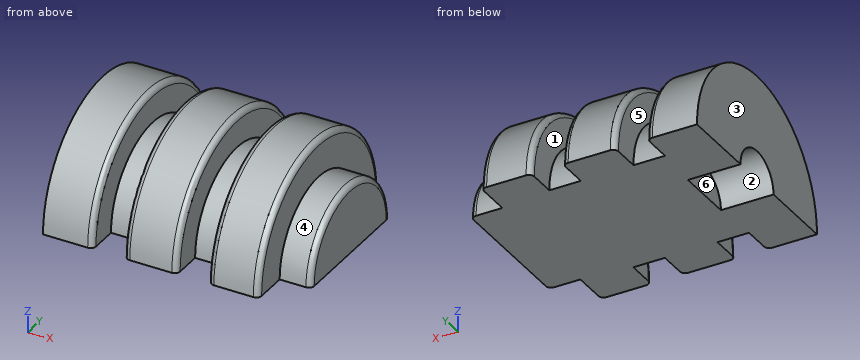
```python
from build123d import *

# Parameters (mm, degrees)
SKETCH1_R           = 10
BOSS_EXTRUDE1_DEPTH = 4.75
SKETCH4_R           = 6.5
BOSS_EXTRUDE2_DEPTH = 3
SKETCH5_R           = 7
BOSS_EXTRUDE3_DEPTH = 3
FILLET1_R           = 0.5
BOSS_EXTRUDE4_START = 5
SKETCH6_R           = 10
BOSS_EXTRUDE4_DEPTH = 5
SKETCH7_R           = 7
BOSS_EXTRUDE5_DEPTH = 3
BOSS_EXTRUDE6_START = 4.75
SKETCH9_R           = 10
BOSS_EXTRUDE6_DEPTH = 4.75
FILLET2_R           = 0.5
SKETCH10_W          = 23.933386236
SKETCH10_H          = 20
CUT_EXTRUDE1_DEPTH  = 20
CUT_EXTRUDE2_DEPTH  = 5


with BuildPart() as part:
    # Sketch1 → Boss-Extrude1 (new body)
    with BuildSketch(Plane(origin=(0, 0, 0), x_dir=(0, 0, -1), z_dir=(1, 0, 0))):
        Circle(SKETCH1_R)
    extrude(amount=BOSS_EXTRUDE1_DEPTH)

    # Sketch4 → Boss-Extrude2 (add)
    with BuildSketch(Plane(origin=(4.75, 0, 0), x_dir=(0, 0, -1), z_dir=(1, 0, 0))):
        Circle(SKETCH4_R)
    extrude(amount=BOSS_EXTRUDE2_DEPTH)

    # Sketch5 → Boss-Extrude3 (add)
    with BuildSketch(Plane.ZY):
        with Locations(Location((0, 0, 0), (0, 0, 180))):
            Circle(SKETCH5_R)
    extrude(amount=BOSS_EXTRUDE3_DEPTH)

    # Fillet1
    fillet1_edges = [part.edges().sort_by_distance(p)[0] for p in [
        (7.75, 0, 6.5),
    ]]
    fillet(fillet1_edges, radius=FILLET1_R)

    # Sketch6 → Boss-Extrude4 (add)
    with BuildSketch(Plane.ZY.offset(3).offset(BOSS_EXTRUDE4_START)):
        with Locations(Location((0, 0, 0), (0, 0, 180))):
            Circle(SKETCH6_R)
    extrude(amount=-BOSS_EXTRUDE4_DEPTH)

    # Sketch7 → Boss-Extrude5 (add)
    with BuildSketch(Plane.ZY.offset(8)):
        with Locations(Location((0, 0, 0), (0, 0, 180))):
            Circle(SKETCH7_R)
    extrude(amount=BOSS_EXTRUDE5_DEPTH)

    # Sketch9 → Boss-Extrude6 (add)
    with BuildSketch(Plane.ZY.offset(11).offset(BOSS_EXTRUDE6_START)):
        with Locations(Location((0, 0, 0), (0, 0, 180))):
            Circle(SKETCH9_R)
    extrude(amount=-BOSS_EXTRUDE6_DEPTH)

    # Fillet2
    fillet2_edges = [part.edges().sort_by_distance(p)[0] for p in [
        (-3, 0, 10),
        (-8, 0, 10),
        (0, 0, 10),
        (-11, 0, 10),
        (4.75, 0, 10),
    ]]
    fillet(fillet2_edges, radius=FILLET2_R)

    # Sketch10 → Cut-Extrude1 (cut)
    with BuildSketch(Plane.XY):
        with Locations((-3.783306882, 0)):
            Rectangle(SKETCH10_W, SKETCH10_H)
    extrude(amount=-CUT_EXTRUDE1_DEPTH, mode=Mode.SUBTRACT)

    # Sketch11 → Cut-Extrude2 (cut)
    with BuildSketch(Plane.ZY.offset(15.75)):
        with BuildLine():
            Line((0, 2.75), (0, -2.75))
            ThreePointArc((0, -2.75), (2.75, 0), (0, 2.75))
        make_face()
    extrude(amount=-CUT_EXTRUDE2_DEPTH, mode=Mode.SUBTRACT)


solid = part.part
```
Read the model definition and answer for the solid it produces. Units are mm, in the model's axes. Face numbers are marked on the shaded views. A direction names the side the tool comes from. Round coordinates to 2 decimals unless told otherwise and drop trailing zeros. Write each loop counter-clockwise with the first axis right and the second up, starting at its lowest first coordinate (ties: lowest second). Pieces come first, ordered by that corner, then holes. Notation, with made-up numbers: (-36, 46) -> (-17, 46) arc R24 ccw to (-17, 70) -> close; hole circle Ø9 at (-26.75, 52). An arc over 180 degrees is marked (long way). Answer in a Markdown table with one row per item. Add a question column.
1) Given P1, Ø6, axis at x = -1.5, y = 4.5, coming from the +Z side; P2, Ø3, axis at x = 2.5, y = 3, coming from the +Z side; P3, Ø4, axis at x = -5.5, z = 6.5, coming from the +Y side, each flat-ended and moving along its own axis, determine where each tip first touches the part or whether it passes through.
2) Find section C-C, the plane x = -8.5. Determine the outline of the cut face in (y, z).
3) Find section B-B, the plane x = 5.25. Determine the outline of the cut face in (y, z).
4) Consider line 1 (X direction, y = -4.75, z = 7.5); line 2 (X direction, y = 8.5, z = 5); line 3 (X direction, y = 0.75, z = 6.5). Determine where each line is inside the solid, lowest interval first.
5) Find section A-A, the plane y = 0. Determine the outline of the cut face in (x, z), and give its area (3 significant figures).
6) Determine the mould class of the marked faces 1, 2 and 3 for opening direction X: pulls with the +X half, pulls with the -X half, needs draft (parallel to the pull), parting line crosses it, or undercut.
7) Which of the six approach directions +Z, -Z, +X, -X, +Y, -Y give full straight-line access (tool end or side, diameter ignored) to the marked faces 4, 5 and 6?
8) Find section D-D, the plane x = -13.5. Determine the outline of the cut face in (y, z).
Findings below:
| question | item | result |
|---|---|---|
| 1 | P1 | z = 9.75 |
| 1 | P2 | z = 9.89 |
| 1 | P3 | y = 8.93 |
| 2 | outline | (-7, 0) -> (7, 0) arc R7 ccw to start |
| 3 | outline | (-6.5, 0) -> (6.5, 0) arc R6.5 ccw to start |
| 4 | line 1 | -15.75 to -11, -8 to -3, 0 to 4.75 |
| 4 | line 2 | -15.75 to -11.15, -7.85 to -3.15, 0.15 to 4.6 |
| 4 | line 3 | -15.75 to 4.75 |
| 5 | outline | (-15.75, 2.75) -> (-10.75, 2.75) -> (-10.75, 0) -> (7.75, 0) -> (7.75, 6) arc R0.5 ccw to (7.25, 6.5) -> (4.75, 6.5) -> (4.75, 9.5) arc R0.5 ccw to (4.25, 10) -> (0.5, 10) arc R0.5 ccw to (0, 9.5) -> (0, 7) -> (-3, 7) -> (-3, 9.5) arc R0.5 ccw to (-3.5, 10) -> (-7.5, 10) arc R0.5 ccw to (-8, 9.5) -> (-8, 7) -> (-11, 7) -> (-11, 9.5) arc R0.5 ccw to (-11.5, 10) -> (-15.75, 10) -> close |
| 5 | area | 192 mm² |
| 6 | face 1 | undercut |
| 6 | face 2 | needs draft |
| 6 | face 3 | pulls with the -X half |
| 7 | face 4 | +Z, +X |
| 7 | face 5 | +Z |
| 7 | face 6 | -Z, -X |
| 8 | outline | (-10, 0) -> (-2.75, 0) arc R2.75 cw to (2.75, 0) -> (10, 0) arc R10 ccw to start |
